from build123d import *

# Parameters (mm, degrees)
SKETCH2_R          = 6.125
SKETCH2_R_2        = 4.25
SKETCH2_R_3        = 1.75
EXTRUDE1_DEPTH     = 8
SKETCH3_W          = 8.5
SKETCH3_H          = 15
SKETCH3_W_2        = 15.5
SKETCH3_H_2        = 8.5
EXTRUDE2_DEPTH     = 10
SKETCH4_R          = 2.5
CUT_EXTRUDE1_DEPTH = 169.256392057


with BuildPart() as part:
    # Sketch2 → Extrude1 (new body)
    with BuildSketch(Plane.XY):
        with BuildLine():
            Line((59.608556798, 87.780072478), (59.608556798, 79.780072478))
            Line((59.608556798, 79.780072478), (59.608556798, 64.280072478))
            Line((59.608556798, 64.280072478), (67.315449876, 64.280072478))
            ThreePointArc((67.315449876, 64.280072478), (67.608054466, 64.27150339), (67.899656114, 64.2458255))
            Line((67.899656114, 64.2458255), (131.192763036, 56.799577626))
            ThreePointArc((131.192763036, 56.799577626), (134.344934134, 55.156396561), (135.608556798, 51.833824605))
            Line((135.608556798, 51.833824605), (135.608556798, 6.280072478))
            Line((135.608556798, 6.280072478), (67.608556798, 6.280072478))
            Line((67.608556798, 6.280072478), (59.608556798, 6.280072478))
            Line((59.608556798, 6.280072478), (58.204496826, 6.280072478))
            ThreePointArc((58.204496826, 6.280072478), (55.900569943, 6.842514488), (54.114973167, 8.403304111))
            Line((54.114973167, 8.403304111), (4.972747334, 78.262350637))
            ThreePointArc((4.972747334, 78.262350637), (4.70177693, 78.809575974), (4.608556798, 79.413057984))
            Line((4.608556798, 79.413057984), (4.608556798, 85.309690651))
            ThreePointArc((4.608556798, 85.309690651), (4.997175407, 86.494363608), (6.012006812, 87.218650607))
            Line((6.012006812, 87.218650607), (44.317228657, 99.189032434))
            ThreePointArc((44.317228657, 99.189032434), (44.612050216, 99.257181467), (44.913778644, 99.280072478))
            Line((44.913778644, 99.280072478), (58.608556798, 99.280072478))
            ThreePointArc((58.608556798, 99.280072478), (59.315663579, 98.987179259), (59.608556798, 98.280072478))
            Line((59.608556798, 98.280072478), (59.608556798, 87.780072478))
        make_face()
        with Locations((127.108556798, 37.780072478)):
            Circle(SKETCH2_R, mode=Mode.SUBTRACT)
        with Locations((127.108556798, 14.780072478)):
            Circle(SKETCH2_R_2, mode=Mode.SUBTRACT)
        with Locations((116.501954798, 25.386674196)):
            Circle(SKETCH2_R_3, mode=Mode.SUBTRACT)
        with Locations((63.608556798, 43.780072478)):
            Circle(SKETCH2_R_3, mode=Mode.SUBTRACT)
        with Locations((35.108556798, 83.780072478)):
            Circle(SKETCH2_R_3, mode=Mode.SUBTRACT)
    extrude(amount=EXTRUDE1_DEPTH)

    # Sketch3 → Extrude2 (cut)
    with BuildSketch(Plane.XY.offset(8)):
        with Locations((63.608556798, 13.780072478)):
            Rectangle(SKETCH3_W, SKETCH3_H)
        with Locations((51.858556798, 83.780072478)):
            Rectangle(SKETCH3_W_2, SKETCH3_H_2)
    extrude(amount=-EXTRUDE2_DEPTH, mode=Mode.SUBTRACT)

    # Sketch4 → Cut-Extrude1 (cut, through all)
    with BuildSketch(Plane(origin=(0, 0, 0), x_dir=(-1, 0, 0), z_dir=(0, 0, -1))):
        with Locations((-22.880634737, 69.007994539)):
            Circle(SKETCH4_R)
        with Locations((-48.336478859, 43.552150417)):
            Circle(SKETCH4_R)
    extrude(amount=-CUT_EXTRUDE1_DEPTH, mode=Mode.SUBTRACT)


solid = part.part
For this review, take the finished solid that the model builds, in its own axes (mm). A direction names the side the tool comes from. Round coordinates to 2 decimals unless told otherwise and drop trailing zeros. Write each loop counter-clockwise with the first axis right and the second up, starting at its lowest first coordinate (ties: lowest second). Pieces come first, ordered by that corner, then holes. Notation, with made-up numbers: (65.5, 65) - (78.5, 65) arc R17 cw to (78.5, 70) - close; hole circle Ø1 at (-31.5, -19.5). An arc over 180 degrees is marked (long way). Use a Markdown table: item, result.
Q1. Machinability: for faces 4 (the flat face through (64, 21.28, 4)), 5 (the flat face through (63, 64.28, 4)), 6 (the flat face through (52, 79.53, 4)), which of the approach directions +Z, -Z, +X, -X, +Y, -Y give a long, thin tool a straight path to every point of the face, cutting with its end or side? Answer none if there is none.
Derived:
| item | result |
|---|---|
| face 4 | +Z, -Z, -Y |
| face 5 | +Z, -Z, +X, +Y |
| face 6 | +Z, -Z, +X |
Q2. Clearance check with flat-ended pins moving along their axes: pin 1 (1 mm diameter, centred on y = 74.5, z = 2, fed in from -X); pin 2 (1.5 mm diameter, centred on y = 63, z = 4, fed in from -X); pin 3 (2.5 mm diameter, centred on x = 64, z = 3.5, fed in from -Y). State where each tip first meets the part, or that it passes through.
Derived:
| item | result |
|---|---|
| pin 1 | stops at x = 7.27 |
| pin 2 | stops at x = 15.18 |
| pin 3 | stops at y = 21.28 |
Q3. We need section D-D (x = 96). Give the boundary of the cut face in (y, z).
Derived:
| item | result |
|---|---|
| outline | (6.28, 0) - (60.94, 0) - (60.94, 8) - (6.28, 8) - close |
Q4. Wall thickness on line 1 along X through (y, z) = (13, 7.25); line 2 along X through (y, z) = (18, 3.25); line 3 along Y through (x, z) = (58, 7.25): over which ranges is each line inside the solid? List them lowest first.
Derived:
| item | result |
|---|---|
| line 1 | x = 50.88 to 59.36, 67.86 to 123.25, 130.97 to 135.61 |
| line 2 | x = 47.36 to 59.36, 67.86 to 124.33, 129.88 to 135.61 |
| line 3 | y = 6.28 to 79.53, 88.03 to 99.28 |
Q5. The part is to be moulded in two halves that separate along X. For faces 1 (the flat face through (52, 88.03, 4)), 2 (the flat face through (59.609, 93, 4)), 3 (the cylindrical face through (132.767, 35.434, 3.944)), say which applies: pulls with the +X half, pulls with the -X half, needs draft (parallel to the pull), parting line crosses it, or undercut.
Derived:
| item | result |
|---|---|
| face 1 | needs draft |
| face 2 | pulls with the +X half |
| face 3 | undercut |
Q6. We need section C-C (y = 54.5). Give the boundary of the cut face in (x, z).
Derived:
| item | result |
|---|---|
| outline | (21.69, 0) - (134.84, 0) - (134.84, 8) - (21.69, 8) - close |
Q7. We need section B-B (z = 1.5). State how many separate pieces and enclosed holes the cut face has, plus the area to 3 significant figures.
Derived:
| item | result |
|---|---|
| separate pieces | 1 |
| enclosed holes | 7 |
| area | 6,640 mm2 |
Q8. We need section A-A (y = 33). Give the boundary of the cut face in (x, z).
Derived:
| item | result |
|---|---|
| outline | (36.81, 0) - (123.28, 0) - (123.28, 8) - (36.81, 8) - close; (130.94, 0) - (135.61, 0) - (135.61, 8) - (130.94, 8) - close |
